Autodesk Inventor part; units mm, degrees
ref_plane "YZ Plane" through (0, 0, 0) normal (1, 0, 0) x (0, 1, 0)
ref_plane "XZ Plane" through (0, 0, 0) normal (0, 1, 0) x (-1, 0, 0)
ref_plane "XY Plane" through (0, 0, 0) normal (0, 0, 1) x (1, 0, 0)
sketch "スケッチ1" plane through (0, 0, 0) normal (0, 0, 1) x (1, 0, 0)
  circle A0 centre (0, 0) radius 27.5
  line L0 (0, 27.5) -> (0, 0)
  line L1 (8, 0) -> (19.445271, -19.445602)
  line L2 (0, 0) -> (27.5, 0)
  circle A1 centre (19.445271, -19.445602) radius 5
  circle A2 centre (0, 0) radius 10
  arc A3 (24.316088, -20.574825) -> (0, 10.000005) centre (0.018653, -14.941839) ccw
  line L3 (24.316088, -20.574825) -> (14.574455, -20.574825)
  arc A4 (14.574455, -20.574825) -> (0.517924, -9.986579) centre (1.227526, -23.669106) ccw
  arc A5 (-24.316088, 20.574825) -> (0, -10.000005) centre (-0.018653, 14.941839) ccw
  arc A6 (-14.574455, 20.574825) -> (-0.517924, 9.986579) centre (-1.227526, 23.669106) ccw
  circle A7 centre (-19.445271, 19.445602) radius 5
  point P0 (-0.517924, 9.986579)
  point P1 (0, -10)
  point P2 (0, 10.000005)
  dimension "d4" = 20
  dimension "d0" = 55
  dimension "d1" = 8
  dimension "d2" = 22.56381
  dimension "d3" = 10
  dimension "d5" = 9.74163
  dimension "d9" = 360
sketch "スケッチ1 outline for 押し出し1" plane through (0, 0, 0) normal (0, 0, 1) x (1, 0, 0)
  arc A0 (14.574455, -20.574825) -> (24.316088, -20.574825) centre (19.445271, -19.445602) ccw
  arc A1 (24.316088, -20.574825) -> (0, 10.000005) centre (0.018653, -14.941839) ccw
  arc A2 (0, 10) -> (-0.517924, 9.986579) centre (0, 0) ccw
  arc A3 (-0.517924, 9.986579) -> (-14.574455, 20.574825) centre (-1.227526, 23.669106) cw
  arc A4 (-14.574455, 20.574825) -> (-24.316088, 20.574825) centre (-19.445271, 19.445602) ccw
  arc A5 (-24.316088, 20.574825) -> (0, -10) centre (-0.018659, 14.941837) ccw
  arc A6 (0, -10) -> (0.517924, -9.986579) centre (0, 0) ccw
  arc A7 (0.517924, -9.986579) -> (14.574455, -20.574825) centre (1.227526, -23.669106) cw
extrude "押し出し1" add sketch "スケッチ1 outline for 押し出し1" along normal blind 3
sketch "スケッチ2" plane through (0, 0, 3) normal (0, 0, 1) x (1, 0, 0)
  circle A0 centre (0, 0) radius 4.25
  dimension "d13" = 8.5
extrude "押し出し2" cut sketch "スケッチ2" against normal blind 3
sketch "スケッチ3" plane through (0, 0, 3) normal (0, 0, 1) x (1, 0, 0)
  arc A0 (-14.574455, 20.574825) -> (-24.316088, 20.574825) centre (-19.445271, 19.445602) ccw
  arc A1 (14.574455, -20.574825) -> (24.316088, -20.574825) centre (19.445271, -19.445602) ccw
  circle A2 centre (0, 0) radius 4.25
  point P0 (8, 0)
  point P1 (-8, 0)
  point P2 (0, 8)
  point P3 (-8, 0)
  point P4 (0, -8)
  dimension "d16" = 8
  dimension "d17" = 8
  dimension "d49" = 360
hole "穴1" at (-19.445271, 19.445602, 3) at (19.445271, -19.445602, 3) at (8, 0, 3) at (-8, 0, 3) at (0, 8, 3) at (0, -8, 3) direction (0, 0, -1) diameter 2.3 end through all
sketch "スケッチ4" plane through (0, 0, 3) normal (0, 0, 1) x (1, 0, 0)
  circle A0 centre (0, 0) radius 9.289
  circle A1 centre (8, 0) radius 1.15
  circle A2 centre (8, 0) radius 6.227
  circle A3 centre (0, 0) radius 8.107
  circle A4 centre (8, 0) radius 4.267399
  line L0 (6.969375, 6.141119) -> (6.969547, 4.141119)
  circle A5 centre (6.970301, -6.696881) radius 12.838
  circle A6 centre (0, 0) radius 20.909
  circle A7 centre (8, 0) radius 13.574
  line L1 (19.8083, -6.694589) -> (17.8083, -6.694761)
  arc A8 (17.8083, -6.694761) -> (6.969547, 4.141119) centre (6.970301, -6.696881) ccw
  circle A9 centre (-6.970301, 6.696881) radius 12.838
  line L2 (-19.8083, 6.694589) -> (-17.8083, 6.694761)
  arc A10 (-17.8083, 6.694761) -> (-6.969547, -4.141119) centre (-6.970301, 6.696881) ccw
  line L3 (-6.969375, -6.141119) -> (-6.969547, -4.141119)
  point P0 (6.969547, 4.141119)
  point P1 (-6.969547, -4.141119)
  dimension "d25" = 18.578
  dimension "d26" = 12.454
  dimension "d30" = 41.818
  dimension "d31" = 27.148
  dimension "d27" = 16.214
  dimension "d29" = 25.676
  dimension "d32" = 2
  dimension "d33" = 2
  dimension "d36" = 360
extrude "押し出し3" add sketch "スケッチ4" along normal blind 2 contours A8 A4 A0 | A0 A4 A8 | A4 L0 A0 | A0 A5 A2 A8 A4 | A2 A5 L1 A8 | A9 L2 A10 A0 | A0 A10 L3 picked at (7.717949, 4.165451) picked at (9.179473, 4.022297)
sketch "スケッチ5" plane through (0, 0, 0) normal (0, 0, -1) x (-1, 0, 0)
  circle A0 centre (19.445271, 19.445602) radius 1.15
  circle A1 centre (-19.445271, -19.445602) radius 1.15
  point P0 (0, 0)
hole "穴2" at (-19.445271, 19.445602, 0) at (19.445271, -19.445602, 0) direction (0, 0, 1) diameter 3.2 end through all
sketch "スケッチ6" plane through (0, 0, 3) normal (0, 0, 1) x (1, 0, 0)
  circle A0 centre (-19.445271, 19.445602) radius 1.6
  circle A1 centre (-19.445271, 19.445602) radius 2.25
  circle A2 centre (-19.445271, 19.445602) radius 4
  circle A3 centre (19.445271, -19.445602) radius 1.6
  circle A4 centre (19.445271, -19.445602) radius 2.25
  circle A5 centre (19.445271, -19.445602) radius 4
  point P0 (0, 0)
  dimension "d51" = 4.5
  dimension "d52" = 8
  dimension "d53" = 4.5
  dimension "d54" = 8
extrude "押し出し4" cut sketch "スケッチ6" against normal blind 0.5 contours A2 | A5
fillet "フィレット1" radius 0.5 4 edges at (-21.6953, 19.4456, 2.5) (17.1953, -19.4456, 2.5) (-23.4453, 19.4456, 3) (15.4453, -19.4456, 3)
properties part number "rotor_ver2" material "アルミニウム 6061"
Input: part model. Units: mm. Frame: model coordinates. A direction names the side the tool comes from. Round coordinates to 2 decimals unless told otherwise and drop trailing zeros. Order: outer loops, then holes, each group sorted by start corner. A loop starts at its lowest first (then second) coordinate and runs counter-clockwise, first axis right, second up. Notation, with made-up numbers: (80.25, -32.75) - (108.25, -32.75) arc R23 ccw to (108.25, -19.75) - close; hole circle Ø8 at (-5, -14). An arc over 180 degrees is marked (long way). Use a Markdown table: item, result.
1. Material intervals for probe 1 along Z at (x, y) = (7, 3); probe 2 along X at (y, z) = (-1, 4.25); probe 3 along Y at (x, z) = (-13.5, 4.85), sorted ascending.
Evaluation:
| item | result |
|---|---|
| probe 1 | 0 to 3 |
| probe 2 | -17.25 to -14.6, 16.19 to 18.48 |
| probe 3 | -4.36 to -1.95 |
2. Section C-C on z = 1.85. Return the cut outline in (x, y).
Evaluation:
| item | result |
|---|---|
| outline | (-24.32, 20.57) arc R24.94 ccw to (0, -10) arc R10 ccw to (0.52, -9.99) arc R13.7 cw to (14.57, -20.57) arc R5 ccw to (24.32, -20.57) arc R24.94 ccw to (0, 10) arc R10.01 ccw to (-0.52, 9.99) arc R13.7 cw to (-14.57, 20.57) arc R5 ccw to start; hole circle Ø3.2 at (-19.45, 19.45); hole circle Ø2.3 at (-8, 0); hole circle Ø8.5 at (0, 0); hole circle Ø2.3 at (0, -8); hole circle Ø2.3 at (0, 8); hole circle Ø2.3 at (8, 0); hole circle Ø3.2 at (19.45, -19.45) |
3. Section D-D on y = 0. Return the cut outline in (x, z).
Evaluation:
| item | result |
|---|---|
| outline | (-19.99, 0) - (-9.15, 0) - (-9.15, 3) - (-15.49, 3) - (-15.49, 5) - (-17.92, 5) - (-17.92, 3) - (-19.99, 3) - close; (-6.85, 0) - (-4.25, 0) - (-4.25, 3) - (-6.85, 3) - close; (4.25, 0) - (6.85, 0) - (6.85, 3) - (4.25, 3) - close; (9.15, 0) - (19.99, 0) - (19.99, 3) - (17.92, 3) - (17.92, 5) - (15.49, 5) - (15.49, 3) - (9.15, 3) - close |
4. Section A-A on y = 8. Return the cut outline in (x, z) (3 decimals).
Evaluation:
| item | result |
|---|---|
| outline | (-23.975, 0) - (-1.15, 0) - (-1.15, 3) - (-23.975, 3) - close; (1.15, 0) - (9.805, 0) - (9.805, 3) - (1.15, 3) - close |
5. Section B-B on x = 3.5. Return the cut outline in (y, z).
Evaluation:
| item | result |
|---|---|
| outline | (-10.16, 0) - (-2.41, 0) - (-2.41, 3) - (-10.16, 3) - close; (2.41, 0) - (9.76, 0) - (9.76, 3) - (2.41, 3) - close |
6. First-contact query: pin 1 (3 mm diameter, centred on y = -2, z = 0.5, fed in from +X); pin 2 (3.5 mm diameter, centred on x = -19.5, y = 18.5, fed in from +Z); pin 3 (0.6 mm diameter, centred on x = 18.5, z = 4, fed in from -Y). Flat tips, straight axial feed; report the tip coordinate or a pass-through.
Evaluation:
| item | result |
|---|---|
| pin 1 | x = 22.18 |
| pin 2 | z = 3 |
| pin 3 | y = -6.69 |
7. Access query for faces 1 (the face through (-20.4, 22.2, 2.5)), 2 (the face through (-15, -1, 5)), 3 (the face through (-14.5, -1.1, 4)), 4 (the face through (-15.95, -2.48, 3.99)). Directions: +Z, -Z, +X, -X, +Y, -Y. A direction counts if a zero-diameter tool reaches every point of the face in a straight line with its end or side. Return the directions, or none.
Evaluation:
| item | result |
|---|---|
| face 1 | +Z |
| face 2 | +Z, +X, -X, +Y, -Y |
| face 3 | +Z, +Y |
| face 4 | +Z, -X, -Y |
